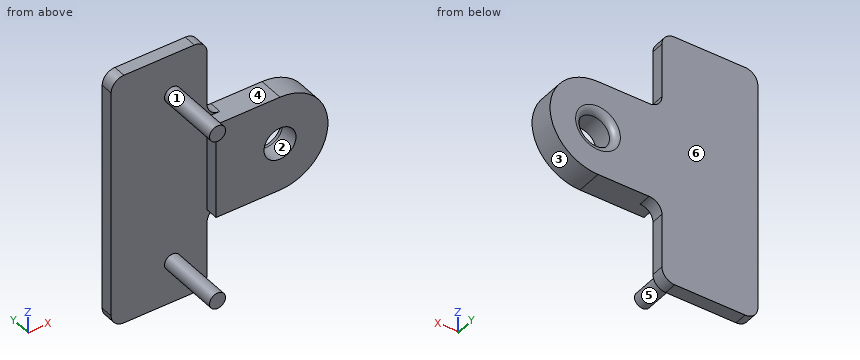
from build123d import *

# Parameters (mm, degrees)
SKETCH_1_W          = 15
SKETCH_1_H          = 40
EXTRUDE_1_DEPTH     = 2
EXTRUDE_2_DEPTH     = 4
SKETCH_3_R          = 1.25
EXTRUDE_3_DEPTH     = 10
CUT_EXTRUDE_1_REACH = 36.191
SKETCH_4_R          = 2.5
FILLET_2_R          = 1
FILLET_3_R          = 2


with BuildPart() as part:
    # 草图1 → 凸台-拉伸1 (new body)
    with BuildSketch(Plane(origin=(0, 0, 0), x_dir=(1, 0, 0), z_dir=(0, 1, 0))):
        Rectangle(SKETCH_1_W, SKETCH_1_H)
    extrude(amount=EXTRUDE_1_DEPTH)

    # 草图2 → 凸台-拉伸2 (add)
    with BuildSketch(Plane(origin=(0, 2, 0), x_dir=(1, 0, 0), z_dir=(0, 1, 0))):
        with BuildLine():
            Line((7.5, -7.5), (17.5, -7.5))
            ThreePointArc((17.5, -7.5), (25, 0), (17.5, 7.5))
            Line((17.5, 7.5), (7.5, 7.5))
            Line((7.5, 7.5), (7.5, -7.5))
        make_face()
    extrude(amount=-EXTRUDE_2_DEPTH)

    # 草图3 → 凸台-拉伸3 (add)
    with BuildSketch(Plane.XZ):
        with Locations(Location((2.1, 13.5, 0), (0, 0, 270))):
            Circle(SKETCH_3_R)
        with Locations(Location((2.1, -13.5, 0), (0, 0, 90))):
            Circle(SKETCH_3_R)
    extrude(amount=EXTRUDE_3_DEPTH)

    # 草图4 → 切除-拉伸1 (cut, up to next)
    with BuildSketch(Plane(origin=(0, 2, 0), x_dir=(1, 0, 0), z_dir=(0, 1, 0)), mode=Mode.PRIVATE) as cut_extrude_1_sk1:
        with Locations(Location((17.5, 0, 0), (0, 0, 270))):
            Circle(SKETCH_4_R)
    cut_extrude_1_tool1 = extrude(cut_extrude_1_sk1.sketch, amount=-CUT_EXTRUDE_1_REACH, mode=Mode.PRIVATE) & part.part
    add(cut_extrude_1_tool1.solids().sort_by_distance((17.5, 2, 0))[0], mode=Mode.SUBTRACT)

    # 圆角2
    fillet_2_edges = [part.edges().sort_by_distance(p)[0] for p in [
        (17.5, 2, -2.5),
    ]]
    fillet(fillet_2_edges, radius=FILLET_2_R)

    # 圆角3
    fillet_3_edges = [part.edges().sort_by_distance(p)[0] for p in [
        (7.5, 1, 7.5),
        (7.5, 1, -7.5),
        (7.5, 1, 20),
        (-7.5, 1, 20),
        (-7.5, 1, -20),
        (7.5, 1, -20),
    ]]
    fillet(fillet_3_edges, radius=FILLET_3_R)


solid = part.part
Model file for the job. Use its own axes, mm. Face numbers are marked on the shaded views. A direction names the side the tool comes from. Round coordinates to 2 decimals unless told otherwise and drop trailing zeros. Loops run counter-clockwise (first coordinate to the right, second up) from the corner with the lowest first, then second, coordinate; pieces in that order, holes last. Notation, with made-up numbers: (43.25, 68.25) - (48.25, 68.25) arc R11 cw to (48.25, 80.25) - close; hole circle Ø3 at (67.25, -20.5). An arc over 180 degrees is marked (long way). Write each question's results on one line, items separated by ' | '.
(1) Saw through at C-C, the plane x = 2.1. List the corners of the cut face in (y, z).
Answer below:
outline: (-10, -14.75) - (0, -14.75) - (0, -20) - (2, -20) - (2, 20) - (0, 20) - (0, 14.75) - (-10, 14.75) - (-10, 12.25) - (0, 12.25) - (0, -12.25) - (-10, -12.25) - close
(2) Mould opens along Z. For the marked faces 3, 4, 5 and 6 say: released by +Z, released by -Z, zero draft, split by the parting line, or undercut.
Answer below:
face 3: split by the parting line | face 4: released by +Z | face 5: undercut | face 6: zero draft
(3) Saw through at A-A, the plane z = 0. List the corners of the cut face in (x, y).
Answer below:
outline: (-7.5, 0) - (7.5, 0) - (7.5, -2) - (15, -2) - (15, 1) arc R1 ccw to (14, 2) - (-7.5, 2) - close; (20, -2) - (25, -2) - (25, 2) - (21, 2) arc R1 ccw to (20, 1) - close
(4) Pin check, flat tips, straight feed: pin 1 (3 mm diameter, centred on x = 12, y = 0, fed in from +Z); pin 2 (1 mm diameter, centred on y = 1, z = 12.5, fed in from +X); pin 3 (2 mm diameter, centred on x = 10.5, y = 0.5, fed in from -Z); pin 4 (4 mm diameter, centred on x = 17.5, z = 0, fed in from -Y). Stop position of each tip, or through.
Answer below:
pin 1: stops at z = 7.5 | pin 2: stops at x = 7.5 | pin 3: stops at z = -7.5 | pin 4: passes through
(5) 3-axis set-ups, long thin cutter, end or side, ignore diameter. For the marked faces 1 and 2: which of +Z, -Z, +X, -X, +Y, -Y reach the whole face in a straight line?
Answer below:
face 1: -Y | face 2: +Y, -Y
(6) Saw through at D-D, the plane z = -13.5. List the corners of the cut face in (x, y), then the cut area to 3 significant figures.
Answer below:
outline: (-7.5, 0) - (0.85, 0) - (0.85, -10) - (3.35, -10) - (3.35, 0) - (7.5, 0) - (7.5, 2) - (-7.5, 2) - close | area: 55.0 mm^2
(7) Saw through at B-B, the plane y = -1. List the corners of the cut face in (x, z).
Answer below:
outline: circle Ø2.5 at (2.1, -13.5); circle Ø2.5 at (2.1, 13.5); (7.5, -7.5) - (17.5, -7.5) arc R7.5 ccw to (17.5, 7.5) - (7.5, 7.5) - close; hole circle Ø5 at (17.5, 0)
(8) Wall check: L1, parallel to X at y = 0.35, z = 0; L2, parallel to X at y = -0.5, z = 0; L3, parallel to Z at x = 2, y = -9. Give the ranges that are in metal, low to high.
Answer below:
L1: x = -7.5 to 15, 20 to 25 | L2: x = 7.5 to 15, 20 to 25 | L3: z = -14.75 to -12.25, 12.25 to 14.75
